Verification items for the finished model (mm, model axes). Face numbers are marked on the shaded views. Round coordinates to 2 decimals unless told otherwise and drop trailing zeros. Order: outer loops, then holes, each group sorted by start corner. A loop starts at its lowest first (then second) coordinate and runs counter-clockwise, first axis right, second up. Notation, with made-up numbers: M 4.5,9 L 34.5,9 A13 ccw 34.5,24 Z; hole C -29.75,47.25 d3. An arc over 180 degrees is marked long. One line per item, written item: value. Start each with the question number.
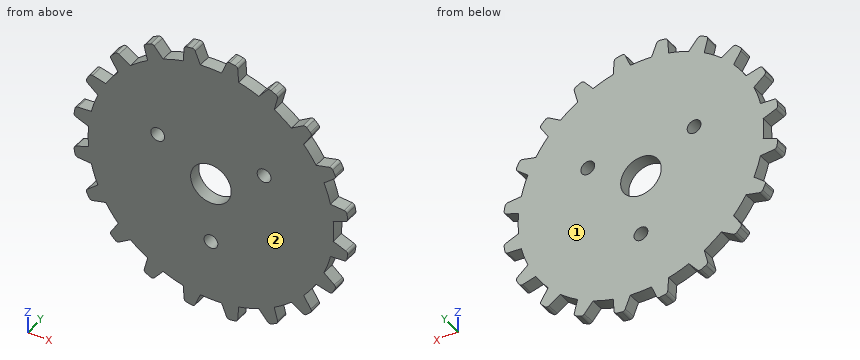
from build123d import *

# Parameters (mm, degrees)
BOSS_EXTRUDE1_DEPTH = 2.5
FILLET1_R           = 0.6
SKETCH5_R           = 1.35
CUT_EXTRUDE4_DEPTH  = 3.5
SKETCH6_R           = 3.96875
CUT_EXTRUDE5_DEPTH  = 3.5


with BuildPart() as part:
    # Sketch1 → Boss-Extrude1 (new body)
    with BuildSketch(Plane(origin=(0, 0, 0), x_dir=(1, 0, 0), z_dir=(0, 1, 0))):
        with BuildLine():
            Line((-2.069685574, 23.903244449), (-3.232226288, 26.798460531))
            ThreePointArc((-3.232226288, 26.798460531), (-4.222590109, 26.66035458), (-5.207159099, 26.485661549))
            Line((-5.207159099, 26.485661549), (-5.418128963, 23.372902518))
            ThreePointArc((-5.418128963, 23.372902518), (-7.414149843, 22.818393363), (-9.354896707, 22.093768379))
            Line((-9.354896707, 22.093768379), (-11.3552096, 24.488037662))
            ThreePointArc((-11.3552096, 24.488037662), (-12.25442448, 24.050651847), (-13.136822119, 23.580260351))
            Line((-13.136822119, 23.580260351), (-12.375570942, 20.554657318))
            ThreePointArc((-12.375570942, 20.554657318), (-14.102546855, 19.410483399), (-15.724385372, 18.121600323))
            Line((-15.724385372, 18.121600323), (-18.36666588, 19.780555048))
            ThreePointArc((-18.36666588, 19.780555048), (-19.086710402, 19.086703739), (-19.78056146, 18.366658976))
            Line((-19.78056146, 18.366658976), (-18.121605812, 15.724379046))
            ThreePointArc((-18.121605812, 15.724379046), (-19.410488322, 14.102540079), (-20.554661637, 12.375563767))
            Line((-20.554661637, 12.375563767), (-23.580264936, 13.136813888))
            ThreePointArc((-23.580264936, 13.136813888), (-24.050656124, 12.254416085), (-24.488041625, 11.355201052))
            Line((-24.488041625, 11.355201052), (-22.093771644, 9.354888995))
            ThreePointArc((-22.093771644, 9.354888995), (-22.818395951, 7.414141878), (-23.37290441, 5.418120804))
            Line((-23.37290441, 5.418120804), (-26.485663367, 5.207149854))
            ThreePointArc((-26.485663367, 5.207149854), (-26.660356054, 4.222580803), (-26.798461659, 3.232216933))
            Line((-26.798461659, 3.232216933), (-23.903245172, 2.06967723))
            ThreePointArc((-23.903245172, 2.06967723), (-23.99268, -4.188e-06), (-23.903244449, -2.069685574))
            Line((-23.903244449, -2.069685574), (-26.798460531, -3.232226288))
            ThreePointArc((-26.798460531, -3.232226288), (-26.66035458, -4.222590109), (-26.485661549, -5.207159099))
            Line((-26.485661549, -5.207159099), (-23.372902518, -5.418128963))
            ThreePointArc((-23.372902518, -5.418128963), (-22.818393363, -7.414149843), (-22.093768379, -9.354896707))
            Line((-22.093768379, -9.354896707), (-24.488037662, -11.3552096))
            ThreePointArc((-24.488037662, -11.3552096), (-24.050651847, -12.25442448), (-23.580260351, -13.136822119))
            Line((-23.580260351, -13.136822119), (-20.554657318, -12.375570942))
            ThreePointArc((-20.554657318, -12.375570942), (-19.410483399, -14.102546855), (-18.121600323, -15.724385372))
            Line((-18.121600323, -15.724385372), (-19.780555048, -18.36666588))
            ThreePointArc((-19.780555048, -18.36666588), (-19.086703739, -19.086710402), (-18.366658976, -19.78056146))
            Line((-18.366658976, -19.78056146), (-15.724379046, -18.121605812))
            ThreePointArc((-15.724379046, -18.121605812), (-14.102540079, -19.410488322), (-12.375563767, -20.554661637))
            Line((-12.375563767, -20.554661637), (-13.136813888, -23.580264936))
            ThreePointArc((-13.136813888, -23.580264936), (-12.254416085, -24.050656124), (-11.355201052, -24.488041625))
            Line((-11.355201052, -24.488041625), (-9.354888995, -22.093771644))
            ThreePointArc((-9.354888995, -22.093771644), (-7.414141878, -22.818395951), (-5.418120804, -23.37290441))
            Line((-5.418120804, -23.37290441), (-5.207149854, -26.485663367))
            ThreePointArc((-5.207149854, -26.485663367), (-4.222580803, -26.660356054), (-3.232216933, -26.798461659))
            Line((-3.232216933, -26.798461659), (-2.06967723, -23.903245172))
            ThreePointArc((-2.06967723, -23.903245172), (4.188e-06, -23.99268), (2.069685574, -23.903244449))
            Line((2.069685574, -23.903244449), (3.232226288, -26.798460531))
            ThreePointArc((3.232226288, -26.798460531), (4.222590109, -26.66035458), (5.207159099, -26.485661549))
            Line((5.207159099, -26.485661549), (5.418128963, -23.372902518))
            ThreePointArc((5.418128963, -23.372902518), (7.414149843, -22.818393363), (9.354896707, -22.093768379))
            Line((9.354896707, -22.093768379), (11.3552096, -24.488037662))
            ThreePointArc((11.3552096, -24.488037662), (12.25442448, -24.050651847), (13.136822119, -23.580260351))
            Line((13.136822119, -23.580260351), (12.375570942, -20.554657318))
            ThreePointArc((12.375570942, -20.554657318), (14.102546855, -19.410483399), (15.724385372, -18.121600323))
            Line((15.724385372, -18.121600323), (18.36666588, -19.780555048))
            ThreePointArc((18.36666588, -19.780555048), (19.086710402, -19.086703739), (19.78056146, -18.366658976))
            Line((19.78056146, -18.366658976), (18.121605812, -15.724379046))
            ThreePointArc((18.121605812, -15.724379046), (19.410488322, -14.102540079), (20.554661637, -12.375563767))
            Line((20.554661637, -12.375563767), (23.580264936, -13.136813888))
            ThreePointArc((23.580264936, -13.136813888), (24.050656124, -12.254416085), (24.488041625, -11.355201052))
            Line((24.488041625, -11.355201052), (22.093771644, -9.354888995))
            ThreePointArc((22.093771644, -9.354888995), (22.818395951, -7.414141878), (23.37290441, -5.418120804))
            Line((23.37290441, -5.418120804), (26.485663367, -5.207149854))
            ThreePointArc((26.485663367, -5.207149854), (26.660356054, -4.222580803), (26.798461659, -3.232216933))
            Line((26.798461659, -3.232216933), (23.903245172, -2.06967723))
            ThreePointArc((23.903245172, -2.06967723), (23.99268, 4.188e-06), (23.903244449, 2.069685574))
            Line((23.903244449, 2.069685574), (26.798460531, 3.232226288))
            ThreePointArc((26.798460531, 3.232226288), (26.66035458, 4.222590109), (26.485661549, 5.207159099))
            Line((26.485661549, 5.207159099), (23.372902518, 5.418128963))
            ThreePointArc((23.372902518, 5.418128963), (22.818393363, 7.414149843), (22.093768379, 9.354896707))
            Line((22.093768379, 9.354896707), (24.488037662, 11.3552096))
            ThreePointArc((24.488037662, 11.3552096), (24.050651847, 12.25442448), (23.580260351, 13.136822119))
            Line((23.580260351, 13.136822119), (20.554657318, 12.375570942))
            ThreePointArc((20.554657318, 12.375570942), (19.410483399, 14.102546855), (18.121600323, 15.724385372))
            Line((18.121600323, 15.724385372), (19.780555048, 18.36666588))
            ThreePointArc((19.780555048, 18.36666588), (19.086703739, 19.086710402), (18.366658976, 19.78056146))
            Line((18.366658976, 19.78056146), (15.724379046, 18.121605812))
            ThreePointArc((15.724379046, 18.121605812), (14.102540079, 19.410488322), (12.375563767, 20.554661637))
            Line((12.375563767, 20.554661637), (13.136813888, 23.580264936))
            ThreePointArc((13.136813888, 23.580264936), (12.254416085, 24.050656124), (11.355201052, 24.488041625))
            Line((11.355201052, 24.488041625), (9.354888995, 22.093771644))
            ThreePointArc((9.354888995, 22.093771644), (7.414141878, 22.818395951), (5.418120804, 23.37290441))
            Line((5.418120804, 23.37290441), (5.207149854, 26.485663367))
            ThreePointArc((5.207149854, 26.485663367), (4.222580803, 26.660356054), (3.232216933, 26.798461659))
            Line((3.232216933, 26.798461659), (2.06967723, 23.903245172))
            ThreePointArc((2.06967723, 23.903245172), (-4.188e-06, 23.99268), (-2.069685574, 23.903244449))
        make_face()
    extrude(amount=-BOSS_EXTRUDE1_DEPTH)

    # Fillet1
    fillet1_edges = [part.edges().sort_by_distance(p)[0] for p in [
        (3.232216933, -1.25, -26.798461659),
        (5.207149854, -1.25, -26.485663367),
        (11.355201052, -1.25, -24.488041625),
        (13.136813888, -1.25, -23.580264936),
        (18.366658976, -1.25, -19.78056146),
        (19.780555048, -1.25, -18.36666588),
        (23.580260351, -1.25, -13.136822119),
        (24.488037662, -1.25, -11.3552096),
        (26.485661549, -1.25, -5.207159099),
        (26.798460531, -1.25, -3.232226288),
        (26.798461659, -1.25, 3.232216933),
        (26.485663367, -1.25, 5.207149854),
        (24.488041625, -1.25, 11.355201052),
        (23.580264936, -1.25, 13.136813888),
        (19.78056146, -1.25, 18.366658976),
        (18.36666588, -1.25, 19.780555048),
        (13.136822119, -1.25, 23.580260351),
        (11.3552096, -1.25, 24.488037662),
        (5.207159099, -1.25, 26.485661549),
        (3.232226288, -1.25, 26.798460531),
        (-3.232216933, -1.25, 26.798461659),
        (-5.207149854, -1.25, 26.485663367),
        (-11.355201052, -1.25, 24.488041625),
        (-13.136813888, -1.25, 23.580264936),
        (-18.366658976, -1.25, 19.78056146),
        (-19.780555048, -1.25, 18.36666588),
        (-23.580260351, -1.25, 13.136822119),
        (-24.488037662, -1.25, 11.3552096),
        (-26.485661549, -1.25, 5.207159099),
        (-26.798460531, -1.25, 3.232226288),
        (-26.798461659, -1.25, -3.232216933),
        (-26.485663367, -1.25, -5.207149854),
        (-24.488041625, -1.25, -11.355201052),
        (-23.580264936, -1.25, -13.136813888),
        (-19.78056146, -1.25, -18.366658976),
        (-18.36666588, -1.25, -19.780555048),
        (-13.136822119, -1.25, -23.580260351),
        (-11.3552096, -1.25, -24.488037662),
        (-5.207159099, -1.25, -26.485661549),
        (-3.232226288, -1.25, -26.798460531),
    ]]
    fillet(fillet1_edges, radius=FILLET1_R)

    # Sketch5 → Cut-Extrude4 (cut, through all)
    with BuildSketch(Plane(origin=(0, 0, 0), x_dir=(1, 0, 0), z_dir=(0, 1, 0))):
        with Locations((0, 12)):
            Circle(SKETCH5_R)
        with Locations((10.392304845, -6)):
            Circle(SKETCH5_R)
        with Locations((-10.392304845, -6)):
            Circle(SKETCH5_R)
    extrude(amount=-CUT_EXTRUDE4_DEPTH, mode=Mode.SUBTRACT)

    # Sketch6 → Cut-Extrude5 (cut, through all)
    with BuildSketch(Plane(origin=(0, 0, 0), x_dir=(1, 0, 0), z_dir=(0, 1, 0))):
        Circle(SKETCH6_R)
    extrude(amount=-CUT_EXTRUDE5_DEPTH, mode=Mode.SUBTRACT)


solid = part.part
1. Depth check by flat-ended pin: pin 1 (1 mm diameter, centred on x = -15.5, y = -1.5, fed in from -Z); pin 2 (4.5 mm diameter, centred on x = 0, z = -12, fed in from -Y); pin 3 (1 mm diameter, centred on y = -2, z = 11, fed in from -X). Enter the tip coordinate at first touch or a pass-through.
2. Scan lines: line 1 along Z through (x, y) = (19, -1.75); line 2 along X through (y, z) = (-0.95, 6). Record each from-to range of solid material in increasing order.
3. Draft check along Y on the marked faces 1 and 2. Enter one of: released by +Y, released by -Y, zero draft, split by the parting line, or undercut.
4. Section check A-A (z = 0). Record the cut outline in (x, y).
5. Section check D-D (z = 14). Record the cut outline in (x, y), and give its area (3 significant figures).
6. Section check C-C (y = -0.4). Give the number of separate pieces and of enclosed holes in the cut face, and give its area (3 significant figures).
7. Section check B-B (x = 0). Record the cut outline in (y, z).
Geometry check:
1. pin 1: stops at z = -18.73
1. pin 2: stops at y = -2.5
1. pin 3: stops at x = -24.35
2. line 1: z = -19.17 to -17.12, -14.65 to 14.65, 17.12 to 19.17
2. line 2: x = -23.23 to -11.74, -9.04 to 9.04, 11.74 to 23.23
3. face 1: released by +Y
3. face 2: released by -Y
4. outline: M -23.99,-2.5 L -3.97,-2.5 L -3.97,0 L -23.99,0 Z; M 3.97,-2.5 L 23.99,-2.5 L 23.99,0 L 3.97,0 Z
5. outline: M -19.48,-2.5 L 19.48,-2.5 L 19.48,0 L -19.48,0 Z
5. area: 97.4 mm²
6. separate pieces: 1
6. enclosed holes: 4
6. area: 1,900 mm²
7. outline: M -2.5,-23.99 L 0,-23.99 L 0,-13.35 L -2.5,-13.35 Z; M -2.5,-10.65 L 0,-10.65 L 0,-3.97 L -2.5,-3.97 Z; M -2.5,3.97 L 0,3.97 L 0,23.99 L -2.5,23.99 Z
